Build history of the part. All positions in model axes, mm. A direction names the side the tool comes from. Give positions to 0.01 mm unless a question says otherwise; leave off trailing zeros. Order: outer loops, then holes, each group sorted by start corner. A loop starts at its lowest first (then second) coordinate and runs counter-clockwise, first axis right, second up. Notation, with made-up numbers: M 19.5,-16.75 L 59.5,-16.75 A21 cw 59.5,-1.75 Z; hole C 68.25,-8 d7. An arc over 180 degrees is marked long. One line per item, written item: value.
from build123d import *

# Parameters (mm, degrees)
F0_W     = 6.35
F0_H     = 30.1625
F1_DEPTH = 7.874
F2_W     = 69.596
F2_H     = 28.575
F3_DEPTH = 3.175
F5_DEPTH = 12.7


with BuildPart() as f1:
    # F0 (on Top) → F1 (new body, symmetric)
    with BuildSketch(Plane.XY):
        with Locations((3.175, 29.36875)):
            Rectangle(F0_W, F0_H)
        Polygon((6.35, 14.2875), (0, 14.2875), (0, -14.2875), (6.35, -14.2875), (69.596, -14.2875), (69.596, 14.2875), align=None)
        Polygon((104.648, 44.45), (6.35, 44.45), (6.35, 14.2875), (69.596, 14.2875), align=None)
        with BuildLine():
            ThreePointArc((30.226, 24.638), (24.638484, 30.299565), (30.373118, 35.812063))
            Line((30.373118, 35.812063), (53.954882, 35.812063))
            ThreePointArc((53.954882, 35.812063), (59.689516, 30.299565), (54.102, 24.638))
            Line((54.102, 24.638), (30.226, 24.638))
        make_face(mode=Mode.SUBTRACT)
        with Locations((3.175, -29.36875)):
            Rectangle(F0_W, F0_H)
        Polygon((69.596, -14.2875), (6.35, -14.2875), (6.35, -44.45), (104.648, -44.45), align=None)
        with BuildLine():
            ThreePointArc((30.373118, -35.812063), (24.638484, -30.299565), (30.226, -24.638))
            Line((30.226, -24.638), (54.102, -24.638))
            ThreePointArc((54.102, -24.638), (59.689516, -30.299565), (53.954882, -35.812063))
            Line((53.954882, -35.812063), (30.373118, -35.812063))
        make_face(mode=Mode.SUBTRACT)
    extrude(amount=F1_DEPTH, both=True)

    # F2 (on face) → F3 (join, symmetric)
    with BuildSketch(Plane.XY.offset(7.874)):
        with Locations((34.798, 0)):
            Rectangle(F2_W, F2_H)
    extrude(amount=F3_DEPTH, both=True)

    # F4 (on Top) → F5 (join, symmetric)
    with BuildSketch(Plane.XY):
        Polygon((104.648, 44.45), (69.596, 44.45), (69.596, 26.924), (84.280943, 26.924), align=None)
        Polygon((84.280943, -26.924), (69.596, -26.924), (69.596, -44.45), (104.648, -44.45), align=None)
    extrude(amount=F5_DEPTH, both=True)


solid = f1.part
1) Saw through at A-A, the plane z = 1. Write the cut outline in (x, y), then the cut area to 3 significant figures.
Check values:
outline: M 0,-44.45 L 104.65,-44.45 L 69.6,-14.29 L 69.6,14.29 L 104.65,44.45 L 0,44.45 Z; hole M 30.23,-24.64 A5.59 ccw long 30.37,-35.81 L 53.95,-35.81 A5.59 ccw long 54.1,-24.64 Z; hole M 30.23,24.64 L 54.1,24.64 A5.59 ccw long 53.95,35.81 L 30.37,35.81 A5.59 ccw long Z
area: 6,510 mm^2
2) Mould opens along Y. For faces 5 (the face through (77, 26.924, -10)), 6 (the face through (65, 44.45, 0)), 7 (the face through (83, 38, -12.7)) say: released by +Y, released by -Y, zero draft, split by the parting line, or undercut.
Check values:
face 5: undercut
face 6: released by +Y
face 7: zero draft
3) Saw through at B-B, the plane x = 79. Write the cut outline in (y, z).
Check values:
outline: M -44.45,-12.7 L -26.92,-12.7 L -26.92,-7.87 L -22.38,-7.87 L -22.38,7.87 L -26.92,7.87 L -26.92,12.7 L -44.45,12.7 Z; M 22.38,-7.87 L 26.92,-7.87 L 26.92,-12.7 L 44.45,-12.7 L 44.45,12.7 L 26.92,12.7 L 26.92,7.87 L 22.38,7.87 Z
4) Pin check, flat tips, straight feed: pin 1 (6 mm diameter, centred on y = -30, z = 5, fed in from +X); pin 2 (2.5 mm diameter, centred on y = 34.5, z = -9.5, fed in from -X); pin 3 (2 mm diameter, centred on x = 20, y = 17.5, fed in from +Z). Stop position of each tip, or through.
Check values:
pin 1: x = 91.34
pin 2: x = 69.6
pin 3: z = 7.87
5) Saw through at C-C, the plane x = 65. Write the cut outline in (y, z).
Check values:
outline: M -44.45,-7.87 L 44.45,-7.87 L 44.45,7.87 L 14.29,7.87 L 14.29,11.05 L -14.29,11.05 L -14.29,7.87 L -44.45,7.87 Z
6) Drill centre lines: probe 1 along Y at (x, z) = (43, -6.5); probe 2 along Z at (x, y) = (65, -38.5); probe 3 along X at (y, z) = (-10, 3.5). Where is each one in solid material? Low to high. Write a range as from..to.
Check values:
probe 1: -44.45..-35.81, -24.64..24.64, 35.81..44.45
probe 2: -7.87..7.87
probe 3: 0..69.6
7) Tool access for faces 1 (the face through (34, -14.288, 9)), 2 (the face through (77, 26.924, 10)), 3 (the face through (34, 14.288, 9)), 4 (the face through (69.596, -36, -10)): list every direction of +Z, -Z, +X, -X, +Y, -Y with a clear straight run to the whole face (end or side of a thin tool).
Check values:
face 1: +Z, +X, -X, -Y
face 2: +Z, +X, -X
face 3: +Z, +X, -X, +Y
face 4: -Z, -X, +Y, -Y
8) Saw through at D-D, the plane y = 39. Write the cut outline in (x, z).
Check values:
outline: M 0,-7.87 L 69.6,-7.87 L 69.6,-12.7 L 98.31,-12.7 L 98.31,12.7 L 69.6,12.7 L 69.6,7.87 L 0,7.87 Z
